Source: CAD feature listing. Evaluate the final solid. Frame: model axes, mm. A direction names the side the tool comes from. Round coordinates to 2 decimals unless told otherwise and drop trailing zeros. Write each loop counter-clockwise with the first axis right and the second up, starting at its lowest first coordinate (ties: lowest second). Pieces come first, ordered by that corner, then holes.
Autodesk Fusion 360 part; units mm, degrees
sketch "Sketch1" plane through (0, 0, 0) normal (0, 0, 1) x (1, 0, 0)
  line L0 (-116.1, 70.1) -> (116.1, 70.1) construction
  line L1 (116.1, 70.1) -> (116.1, -70.1) construction
  line L2 (116.1, -70.1) -> (-116.1, -70.1) construction
  line L3 (-116.1, -70.1) -> (-116.1, 70.1) construction
  circle A0 centre (-116.1, 70.1) radius 1.9
  circle A1 centre (-116.1, 0) radius 1.9
  circle A2 centre (-116.1, -70.1) radius 1.9
  circle A3 centre (0, 70.1) radius 1.9
  circle A4 centre (0, -70.1) radius 1.9
  circle A5 centre (116.1, -70.1) radius 1.9
  circle A6 centre (116.1, 0) radius 1.9
  circle A7 centre (116.1, 70.1) radius 1.9
  circle A8 centre (-116.1, 70.1) radius 5.15
  circle A9 centre (-116.1, 0) radius 5.15
  circle A10 centre (-116.1, -70.1) radius 5.15
  circle A11 centre (0, -70.1) radius 5.15
  circle A12 centre (0, 70.1) radius 5.15
  circle A13 centre (116.1, 70.1) radius 5.15
  circle A14 centre (116.1, 0) radius 5.15
  circle A15 centre (116.1, -70.1) radius 5.15
  line L4 (-121.25, 70.1) -> (-121.25, -70.1)
  line L5 (-116.1, -75.25) -> (116.1, -75.25)
  line L6 (121.25, -70.1) -> (121.25, 70.1)
  line L7 (116.1, 75.25) -> (-116.1, 75.25)
  point P0 (0, 70.1)
  point P1 (-116.1, 0)
  dimension "d1" = 232.2
  dimension "d2" = 140.2
  dimension "d3" = 3.8
  dimension "d4" = 3.8
  dimension "d5" = 3.8
  dimension "d6" = 3.8
  dimension "d7" = 3.8
  dimension "d8" = 3.8
  dimension "d9" = 3.8
  dimension "d10" = 3.8
  dimension "d11" = 10.3
  dimension "d12" = 10.3
  dimension "d13" = 10.3
  dimension "d15" = 10.3
  dimension "d16" = 10.3
  dimension "d17" = 10.3
  dimension "d18" = 10.3
  dimension "d19" = 10.3
extrude "Extrude1" add sketch "Sketch1" along normal blind 3 contours A8 | A9 | A11 | A14 | A12 | A8 A10 A13 A15 L4 L5 L6 L7 | A13 | A10 | A15
sketch "Sketch2" plane through (0, 0, 3) normal (0, 0, 1) x (-1, 0, 0)
  circle A0 centre (-116.1, 0) radius 1.9
  circle A1 centre (116.1, -70.1) radius 1.9
  circle A2 centre (-116.1, -70.1) radius 1.9
  circle A3 centre (0, -70.1) radius 1.9
  circle A4 centre (116.1, 0) radius 1.9
  circle A5 centre (0, 70.1) radius 1.9
  circle A6 centre (-116.1, 70.1) radius 1.9
  circle A7 centre (116.1, 70.1) radius 1.9
  line L0 (-116.1, -75.25) -> (116.1, -75.25)
  arc A8 (116.1, -75.25) -> (121.25, -70.1) centre (116.1, -70.1) ccw
  line L1 (121.25, -70.1) -> (121.25, 70.1)
  arc A9 (121.25, 70.1) -> (116.1, 75.25) centre (116.1, 70.1) ccw
  line L2 (116.1, 75.25) -> (-116.1, 75.25)
  arc A10 (-116.1, 75.25) -> (-121.25, 70.1) centre (-116.1, 70.1) ccw
  line L3 (-121.25, 70.1) -> (-121.25, -70.1)
  arc A11 (-121.25, -70.1) -> (-116.1, -75.25) centre (-116.1, -70.1) ccw
  circle A12 centre (116.1, -70.1) radius 5.15
  circle A13 centre (116.1, 0) radius 5.15
  circle A14 centre (116.1, 70.1) radius 5.15
  circle A15 centre (0, -70.1) radius 5.15
  circle A16 centre (-116.1, -70.1) radius 5.15
  circle A17 centre (-116.1, 0) radius 5.15
  circle A18 centre (-116.1, 70.1) radius 5.15
  circle A19 centre (0, 70.1) radius 5.15
  line L4 (116.1, 0) -> (-116.1, 0) construction
  line L5 (0, -70.1) -> (0, 70.1) construction
  circle A20 centre (107.1, -61.1) radius 4
  circle A21 centre (107.1, 61.1) radius 4
  circle A22 centre (-107.1, -61.1) radius 4
  circle A23 centre (-107.1, 61.1) radius 4
  line L6 (116.1, -70.1) -> (116.1, 70.1) construction
  line L7 (116.1, 70.1) -> (-116.1, 70.1) construction
  line L8 (-116.1, 70.1) -> (-116.1, -70.1) construction
  line L9 (-116.1, -70.1) -> (116.1, -70.1) construction
  line L10 (107.1, -65.1) -> (-107.1, -65.1)
  line L11 (-111.1, -61.1) -> (-111.1, 61.1)
  line L12 (-107.1, 65.1) -> (107.1, 65.1)
  line L13 (111.1, -61.1) -> (111.1, 61.1)
  dimension "d22" = 10.3
  dimension "d23" = 10.3
  dimension "d24" = 10.3
  dimension "d25" = 10.3
  dimension "d26" = 10.3
  dimension "d27" = 10.3
  dimension "d28" = 10.3
  dimension "d29" = 10.3
  dimension "d30" = 8
  dimension "d31" = 8
  dimension "d32" = 8
  dimension "d33" = 8
  dimension "d36" = 5
  dimension "d37" = 5
extrude "Extrude4" add sketch "Sketch2" along normal blind 3 contours A13 A15 A17 A19 A20 A21 A22 A23 L10 L11 L12 L13 | A22 | A20 | A23 | A21
equation "d4 = d3"
equation "d5 = d3"
equation "d6 = d3"
equation "d7 = d3"
equation "d8 = d3"
equation "d9 = d3"
equation "d10 = d3"
equation "d12 = d11"
equation "d13 = d11"
equation "d15 = d11"
equation "d16 = d11"
equation "d17 = d11"
equation "d18 = d11"
equation "d19 = d11"
equation "d22 = d11"
equation "d23 = d11"
equation "d24 = d11"
equation "d25 = d11"
equation "d26 = d11"
equation "d27 = d11"
equation "d28 = d11"
equation "d29 = d11"
equation "d31 = d30"
equation "d32 = d30"
equation "d33 = d30"
equation "d37 = d36"
1) Section query B-B on x = 72.5. Return the cut outline in (y, z).
Taken from the geometry:
outline: (-75.25, 0) - (75.25, 0) - (75.25, 3) - (65.1, 3) - (65.1, 6) - (-65.1, 6) - (-65.1, 3) - (-75.25, 3) - close
2) Reachability of faces 1 (the face through (2, -1, 6)), 2 (the face through (-10, -67, 3)) from +Z, -Z, +X, -X, +Y, -Y: full face, straight path, thin tool, end or side. Return the list, or none.
Taken from the geometry:
face 1: +Z, +X, -X, +Y, -Y
face 2: +Z
3) Contact query for flat-ended pins moving along their axis: P1, Ø1.5, axis at y = -39.5, z = 4.5, coming from the -X side; P2, Ø0.9, axis at x = 45.5, z = 4, coming from the +Y side; P3, Ø6, axis at x = -116.1, y = -70.1, coming from the +Z side; P4, Ø3.5, axis at x = 116.1, y = -70.1, coming from the -Z side. Output: stop coordinate, or through.
Taken from the geometry:
P1: stops at x = -111.1
P2: stops at y = 65.1
P3: stops at z = 3
P4: passes through
4) Section query C-C on z = 4.9. Return the cut outline in (x, y).
Taken from the geometry:
outline: (-111.1, -61.1) arc R4 ccw to (-107.1, -65.1) - (-1.23, -65.1) arc R5.15 cw to (1.23, -65.1) - (107.1, -65.1) arc R4 ccw to (111.1, -61.1) - (111.1, -1.23) arc R5.15 cw to (111.1, 1.23) - (111.1, 61.1) arc R4 ccw to (107.1, 65.1) - (1.23, 65.1) arc R5.15 cw to (-1.23, 65.1) - (-107.1, 65.1) arc R4 ccw to (-111.1, 61.1) - (-111.1, 1.23) arc R5.15 cw to (-111.1, -1.23) - close
5) Material intervals for line 1 (Y direction, x = -116.1, z = 1.6); line 2 (X direction, y = 70.1, z = 2.3); line 3 (Y direction, x = 0, z = 1.45), sorted ascending.
Taken from the geometry:
line 1: y = -75.25 to -72, -68.2 to -1.9, 1.9 to 68.2, 72 to 75.25
line 2: x = -121.25 to -118, -114.2 to -1.9, 1.9 to 114.2, 118 to 121.25
line 3: y = -75.25 to -72, -68.2 to 68.2, 72 to 75.25
6) Section query A-A on y = 25.5. Return the cut outline in (x, z).
Taken from the geometry:
outline: (-121.25, 0) - (121.25, 0) - (121.25, 3) - (111.1, 3) - (111.1, 6) - (-111.1, 6) - (-111.1, 3) - (-121.25, 3) - close
